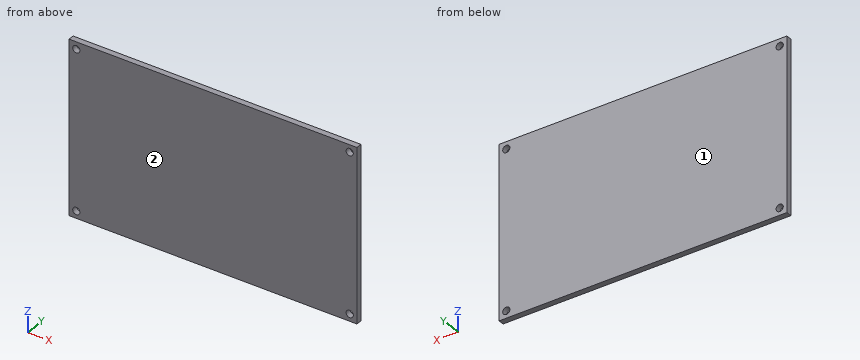
from build123d import *

# Parameters (mm, degrees)
SKETCH2_W                 = 200
SKETCH2_H                 = 120
BOSS_EXTRUDE1_DEPTH       = 4
F_3_0MM_DOWEL_HOLE1_D     = 5
F_3_0MM_DOWEL_HOLE1_DEPTH = 20
F_3_0MM_DOWEL_HOLE1_TIP   = 1.502151548


with BuildPart() as part:
    # Sketch2 → Boss-Extrude1 (new body)
    with BuildSketch(Plane(origin=(0, 0, 0), x_dir=(1, 0, 0), z_dir=(0, 1, 0))):
        Rectangle(SKETCH2_W, SKETCH2_H)
    extrude(amount=BOSS_EXTRUDE1_DEPTH)

    # Ø3.0mm Dowel Hole1
    with Locations(Plane(origin=(-95, 4, -55), x_dir=(0, 0, 1), z_dir=(0, 1, 0))):
        with Locations((0, 0), (110, 0), (110, 190), (0, 190)):
            Hole(F_3_0MM_DOWEL_HOLE1_D / 2, depth=F_3_0MM_DOWEL_HOLE1_DEPTH)
            with Locations((0, 0, -(F_3_0MM_DOWEL_HOLE1_DEPTH + F_3_0MM_DOWEL_HOLE1_TIP / 2))):  # 118° drill point
                Cone(0, F_3_0MM_DOWEL_HOLE1_D / 2, F_3_0MM_DOWEL_HOLE1_TIP, mode=Mode.SUBTRACT)


solid = part.part
Geometry check sheet. Reference: the model listing, model coordinates, mm. Face numbers are marked on the shaded views. Coordinates: 2 decimals unless noted, no trailing zeros. Write each loop counter-clockwise with the first axis right and the second up, starting at its lowest first coordinate (ties: lowest second). Pieces come first, ordered by that corner, then holes. Notation, with made-up numbers: (53.25, -0.5) -> (81.25, -0.5) arc R28 ccw to (81.25, 34.5) -> close; hole circle Ø11 at (25.25, 48.5). An arc over 180 degrees is marked (long way). One line per question, with ' | ' between items.
1. Cross-section at B-B on x = -95. Record the cut outline in (y, z), and give its area (3 significant figures).
Answers:
outline: (0, -60) -> (4, -60) -> (4, -57.5) -> (0, -57.5) -> close; (0, -52.5) -> (4, -52.5) -> (4, 52.5) -> (0, 52.5) -> close; (0, 57.5) -> (4, 57.5) -> (4, 60) -> (0, 60) -> close | area: 440 mm²
2. Cross-section at A-A on z = 55. Record the cut outline in (x, y), and give its area (3 significant figures).
Answers:
outline: (-100, 0) -> (-97.5, 0) -> (-97.5, 4) -> (-100, 4) -> close; (-92.5, 0) -> (92.5, 0) -> (92.5, 4) -> (-92.5, 4) -> close; (97.5, 0) -> (100, 0) -> (100, 4) -> (97.5, 4) -> close | area: 760 mm²
3. Draft check along Y on the marked faces 1 and 2. Enter one of: +Y half, -Y half, draft (parallel to the pull), parting line (faces both ways), or undercut.
Answers:
face 1: +Y half | face 2: -Y half
4. Thickness scan on probe 1 along X at (y, z) = (0.85, -55); probe 2 along X at (y, z) = (2.9, 55.5). Record the ranges inside material, lowest first. Write a range as from..to.
Answers:
probe 1: x = -100..-97.5, -92.5..92.5, 97.5..100 | probe 2: x = -100..-97.45, -92.55..92.55, 97.45..100
